The model under review builds one solid part; all positions refer to its coordinate system, in mm. Face numbers are marked on the shaded views. Coordinates: 2 decimals unless noted, no trailing zeros. Write each loop counter-clockwise with the first axis right and the second up, starting at its lowest first coordinate (ties: lowest second). Pieces come first, ordered by that corner, then holes. Notation, with made-up numbers: (-39.75, 1.5) - (-10.75, 1.5) arc R18 cw to (-10.75, 7.5) - close; hole circle Ø1 at (-4.75, 63). An arc over 180 degrees is marked (long way). Return JSON: item names as keys, results as strings. Group by question number.
(1) We need section D-D on y = 36. State the section outline as (x, z) points.
(2) For pin 1 Ø4 at (y, z) = (13.5, 7.5) entering from -X; pin 2 Ø5.5 at (x, y) = (81, 10.5) entering from +Z, all flat-tipped, find the tip position at first contact; note any pin that passes through.
(3) We need section B-B on x = 81. State the section outline as (y, z) points, then the cut area to 3 significant figures.
(4) Draft analysis for pull direction X (two halves, no side actions). For the marked faces 1, 2 and 3, state which applies: released by +X, released by -X, zero draft, split by the parting line, or undercut.
(5) We need section A-A on z = 5.25. Give the number of separate pieces and of enclosed holes in the cut face, then the cut area to 3 significant figures.
(6) To check wall thickness, follow L1, parallel to Y at x = 43.4, z = 7.25; L2, parallel to Y at x = 17, z = 9.75; L3, parallel to X at y = 11, z = 2 (3 decimals). State the ranges of each line that lie inside material, in increasing order. Write a range as from..to.
```python
from build123d import *

# Parameters (mm, degrees)
F0_R     = 12.5
F1_DEPTH = 10
F2_R     = 8.4
F2_R_2   = 3.3
F2_R_3   = 7.55
F2_R_4   = 3.75
F3_DEPTH = 1
F4_DEPTH = 9


with BuildPart() as f1:
    # F0 (on Top) → F1 (new body)
    with BuildSketch(Plane.XY):
        with BuildLine():
            ThreePointArc((0, 17.5), (5.125631, 5.125631), (17.5, 0))
            Line((17.5, 0), (105, 0))
            ThreePointArc((105, 0), (108.535534, 1.464466), (110, 5))
            Line((110, 5), (110, 35))
            ThreePointArc((110, 35), (108.535534, 38.535534), (105, 40))
            Line((105, 40), (17.5, 40))
            ThreePointArc((17.5, 40), (5.125631, 34.874369), (0, 22.5))
            Line((0, 22.5), (0, 17.5))
        make_face()
        with Locations((17.5, 20)):
            Circle(F0_R, mode=Mode.SUBTRACT)
    extrude(amount=F1_DEPTH)

    # F2 (on face) → F3 (join)
    with BuildSketch(Plane.XY.offset(10)):
        with Locations((43.4, 29.2)):
            Circle(F2_R)
        with Locations((43.4, 29.2)):
            Circle(F2_R_2, mode=Mode.SUBTRACT)
        with Locations((62.2, 29.2)):
            Circle(F2_R)
        with Locations((62.2, 29.2)):
            Circle(F2_R_2, mode=Mode.SUBTRACT)
        with Locations((62.2, 10.4)):
            Circle(F2_R)
        with Locations((62.2, 10.4)):
            Circle(F2_R_2, mode=Mode.SUBTRACT)
        with Locations((43.4, 10.4)):
            Circle(F2_R)
        with Locations((43.4, 10.4)):
            Circle(F2_R_2, mode=Mode.SUBTRACT)
        with Locations((81, 10.4)):
            Circle(F2_R)
        with Locations((81, 10.4)):
            Circle(F2_R_2, mode=Mode.SUBTRACT)
        with Locations((81, 29.2)):
            Circle(F2_R)
        with Locations((81, 29.2)):
            Circle(F2_R_2, mode=Mode.SUBTRACT)
        with Locations((99, 19.8)):
            Circle(F2_R_3)
        with Locations((99, 19.8)):
            Circle(F2_R_4, mode=Mode.SUBTRACT)
    extrude(amount=F3_DEPTH)

    # F2 (on face) → F4 (cut)
    with BuildSketch(Plane.XY.offset(10)):
        with Locations((99, 19.8)):
            Circle(F2_R_4)
        with Locations((81, 29.2)):
            Circle(F2_R_2)
        with Locations((81, 10.4)):
            Circle(F2_R_2)
        with Locations((62.2, 10.4)):
            Circle(F2_R_2)
        with Locations((62.2, 29.2)):
            Circle(F2_R_2)
        with Locations((43.4, 29.2)):
            Circle(F2_R_2)
        with Locations((43.4, 10.4)):
            Circle(F2_R_2)
    extrude(amount=-F4_DEPTH, mode=Mode.SUBTRACT)


solid = f1.part
```
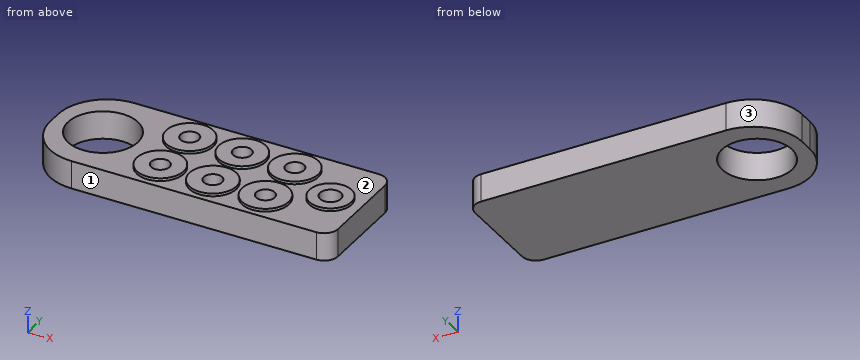
Ans:
{
 "1": {"outline": "(6.36, 0) - (109.9, 0) - (109.9, 10) - (85.93, 10) - (85.93, 11) - (76.07, 11) - (76.07, 10) - (67.13, 10) - (67.13, 11) - (57.27, 11) - (57.27, 10) - (48.33, 10) - (48.33, 11) - (38.47, 11) - (38.47, 10) - (6.36, 10) - close"},
 "2": {"pin 1": "x = 0.11", "pin 2": "z = 1"},
 "3": {"outline": "(0, 0) - (40, 0) - (40, 10) - (37.6, 10) - (37.6, 11) - (32.5, 11) - (32.5, 1) - (25.9, 1) - (25.9, 11) - (20.8, 11) - (20.8, 10) - (18.8, 10) - (18.8, 11) - (13.7, 11) - (13.7, 1) - (7.1, 1) - (7.1, 11) - (2, 11) - (2, 10) - (0, 10) - close", "area": "302 mm²"},
 "4": {"face 1": "zero draft", "face 2": "undercut", "face 3": "released by -X"},
 "5": {"separate pieces": "1", "enclosed holes": "8", "area": "3,520 mm²"},
 "6": {"L1": "0..7.1, 13.7..25.9, 32.5..40", "L2": "0.01..7.51, 32.49..39.99", "L3": "1.252..8.825, 26.175..40.155, 46.645..58.955, 65.445..77.755, 84.245..110"}
}
